Read the model definition and answer for the solid it produces. Units are mm, in the model's axes. Face numbers are marked on the shaded views. Coordinates: 2 decimals unless noted, no trailing zeros. Loops run counter-clockwise (first coordinate to the right, second up) from the corner with the lowest first, then second, coordinate; pieces in that order, holes last.
Q1. Section A-A (y = 0) is taken. Give the vertices of the cut face in (x, z).
Q2. Section C-C (z = -373) is taken. Give the vertices of the cut face in (x, y).
Q3. Flat-ended cylindrical pins translate along their axes: P1, Ø2, axis at y = -59.5, z = -337, coming from the +X side; P2, Ø10, axis at x = 90.5, z = -164.5, coming from the -Y side; P3, Ø5, axis at x = -51.5, z = -303, coming from the +Y side. Find the tip coordinate at first contact, or state that the pin passes through.
Q4. Straight lines are drawn through the part: line 1 (Z direction, x = 102, y = 142.5); line 2 (X direction, y = -78.5, z = -200); line 3 (Y direction, x = 23, z = -309.5). For each, find the intervals that lie inside material, in ascending order.
Q5. The mould has two halves that part along Y. Classify the marked faces 1, 2 and 3: pulls with the +Y half, pulls with the -Y half, needs draft (parallel to the pull), parting line crosses it, or undercut.
Q6. Section D-D (x = -120) is taken. Count the separate pieces of the cut face and the enclosed holes in it, then the cut area to 3 significant figures.
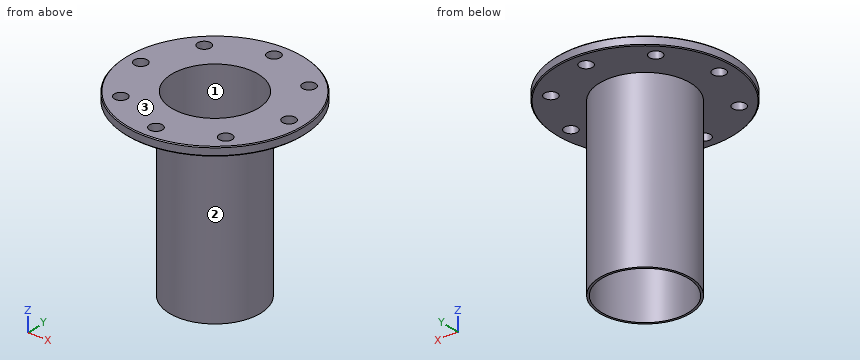
from build123d import *

# Parameters (mm, degrees)
SKETCH2_R          = 15
CUT_EXTRUDE1_DEPTH = 20
CHAMFER1_SIZE      = 2


with BuildPart() as part:
    # Sketch1 → Revolve1 (revolve)
    with BuildSketch(Plane(origin=(0, 0, 0), x_dir=(0, 0, -1), z_dir=(1, 0, 0)), mode=Mode.PRIVATE) as revolve1_sk:
        Polygon((0, 100), (0, 205), (20, 205), (20, 105), (420, 105), (420, 100), align=None)
    revolve(revolve1_sk.sketch.rotate(Axis((0, 0, 0), (0, 0, -1)), 90), axis=Axis((0, 0, 0), (0, 0, -1)))

    # Sketch2 → Cut-Extrude1 (cut)
    with BuildSketch(Plane.XY):
        with Locations((0, 170)):
            Circle(SKETCH2_R)
        with Locations((120.208152802, 120.208152802)):
            Circle(SKETCH2_R)
        with Locations((170, 0)):
            Circle(SKETCH2_R)
        with Locations((120.208152802, -120.208152802)):
            Circle(SKETCH2_R)
        with Locations((0, -170)):
            Circle(SKETCH2_R)
        with Locations((-120.208152802, -120.208152802)):
            Circle(SKETCH2_R)
        with Locations((-170, 0)):
            Circle(SKETCH2_R)
        with Locations((-120.208152802, 120.208152802)):
            Circle(SKETCH2_R)
    extrude(amount=-CUT_EXTRUDE1_DEPTH, mode=Mode.SUBTRACT)

    # Chamfer1
    chamfer1_edges = [part.edges().sort_by_distance(p)[0] for p in [
        (-205, 0, -20),
        (-205, 0, 0),
    ]]
    chamfer(chamfer1_edges, length=CHAMFER1_SIZE)


solid = part.part
Numbers:
1. outline: (-205, -18) - (-203, -20) - (-185, -20) - (-185, 0) - (-203, 0) - (-205, -2) - close; (-155, -20) - (-105, -20) - (-105, -420) - (-100, -420) - (-100, 0) - (-155, 0) - close; (100, -420) - (105, -420) - (105, -20) - (155, -20) - (155, 0) - (100, 0) - close; (185, -20) - (203, -20) - (205, -18) - (205, -2) - (203, 0) - (185, 0) - close
2. outline: circle Ø210 at (0, 0); hole circle Ø200 at (0, 0)
3. P1: stops at x = 87.19
3. P2: stops at y = -60.95
3. P3: stops at y = 92.87
4. line 1: z = -20 to 0
4. line 2: x = -69.73 to -61.95, 61.95 to 69.73
4. line 3: y = -102.45 to -97.32, 97.32 to 102.45
5. face 1: undercut
5. face 2: parting line crosses it
5. face 3: needs draft
6. separate pieces: 3
6. enclosed holes: 0
6. area: 5,440 mm2
